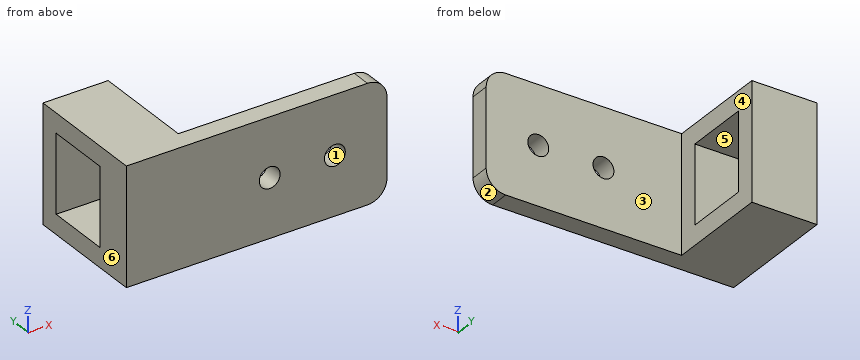
Autodesk Inventor part; units mm, degrees
ref_plane "YZ Plane" through (0, 0, 0) normal (1, 0, 0) x (0, 1, 0)
ref_plane "XZ Plane" through (0, 0, 0) normal (0, 1, 0) x (-1, 0, 0)
ref_plane "XY Plane" through (0, 0, 0) normal (0, 0, 1) x (1, 0, 0)
sketch "Sketch1" plane through (0, 0, 0) normal (1, 0, 0) x (0, 1, 0)
  line L0 (0, 0) -> (10, 0)
  line L1 (10, 0) -> (10, -12)
  line L2 (10, -12) -> (0, -12)
  line L3 (0, -12) -> (0, 0)
  line L4 (13, 3) -> (-6, 3)
  line L5 (-6, 3) -> (-6, -15)
  line L6 (-6, -15) -> (13, -15)
  line L7 (13, -15) -> (13, 3)
  dimension "d0" = 10
  dimension "d1" = 12
  dimension "d2" = 3
  dimension "d3" = 3
  dimension "d4" = 6
  dimension "d5" = 3
extrude "Extrusion1" add sketch "Sketch1" along normal blind 10
sketch "Sketch2" plane through (10, 0, 0) normal (1, 0, 0) x (0, 0, -1)
  line L0 (15, -6) -> (15, 13) construction
  line L1 (-3, -6) -> (15, -6) construction
  line L2 (-3, 13) -> (-3, -6) construction
  line L3 (15, -6) -> (15, 13)
  line L4 (-3, -6) -> (15, -6)
  line L5 (15, -6) -> (15, -3)
  line L6 (15, -3) -> (-3, -3)
  line L7 (-3, -3) -> (-3, -6)
  point P0 (0, 0)
  dimension "d8" = 3
extrude "Extrusion2" add sketch "Sketch2" along normal blind 30
sketch "Sketch3" plane through (10, -3, 3) normal (0, 1, 0) x (1, 0, 0)
  circle A0 centre (12, 9) radius 1.6
  circle A1 centre (22, 9) radius 1.6
  line L0 (0, 18) -> (30, 18)
  line L1 (0, 0) -> (30, 0)
  line L2 (30, 18) -> (30, 0)
  point P0 (-10, 3)
  dimension "d11" = 3.2
  dimension "d12" = 3.2
  dimension "d13" = 9
  dimension "d14" = 9
  dimension "d15" = 8
  dimension "d16" = 10
extrude "Extrusion3" cut sketch "Sketch3" against normal through all
fillet "Fillet1" radius 3 2 edges at (40, -4.5, 3) (40, -4.5, -15)
equation "\"d3\" = d2"
equation "\"d4\" = 2 * d2"
equation "\"d5\" = d2"
properties part number "Wheel Holder Rev 2"
Part model, mm, in its own coordinate system. Face numbers are marked on the shaded views. A direction names the side the tool comes from. Coordinates: 2 decimals unless noted, no trailing zeros. Loops run counter-clockwise (first coordinate to the right, second up) from the corner with the lowest first, then second, coordinate; pieces in that order, holes last. Notation, with made-up numbers: (84, 42) - (104, 42) arc R29 cw to (104, 70) - close; hole circle Ø8 at (82.25, 52.5). An arc over 180 degrees is marked (long way). Write each question's results on one line, items separated by ' | '. Start each with the question number.
Q1. Probe line 1 along X through (y, z) = (-5.3, -6); line 2 along Y through (x, z) = (9.5, -1); line 3 along Z through (x, y) = (32, -4.45). List the from-to ranges inside material, lowest first.
Q2. Which spindle directions (+Z, -Z, +X, -X, +Y, -Y) get a long thin tool onto all of the face, cutting with end or side? Do the marked faces 4, 5 and 6. Say none if no direction does.
Q3. Two-plate mould, pull along X, no slides. Class the marked faces 1, 2 and 3: +X half, -X half, draft (parallel to the pull), parting line (faces both ways), or undercut.
Q4. Drop flat-ended pins along their axis: pin 1 Ø8 at (y, z) = (4, 0) entering from +X; pin 2 Ø1.9 at (x, z) = (22, -6) entering from +Y; pin 3 Ø1 at (x, z) = (29, 0) entering from +Y. Give the stop position or say it passes through.
Q5. Slice it at B-B on y = 3.5. Give the cut face in (x, z).
Q6. Slice it at D-D on x = 32. Give the cut face in (y, z).
Q7. Slice it at C-C on y = -4. Give the cut face in (x, z), and give its area (3 significant figures).
Q8. Slice it at A-A on z = -6. Give the cut face in (x, y), and give its area (3 significant figures).
Answer:
1) line 1: x = 0 to 20.4, 23.6 to 30.4, 33.6 to 40 | line 2: y = -6 to 0, 10 to 13 | line 3: z = -15 to -7.6, -4.4 to 3
2) face 4: +Z, -Z, +X, +Y | face 5: +X, -X | face 6: +Z, -Z, -X, +Y, -Y
3) face 1: undercut | face 2: +X half | face 3: draft
4) pin 1: stops at x = 10 | pin 2: passes through | pin 3: stops at y = -3
5) outline: (0, -15) - (10, -15) - (10, -12) - (0, -12) - close; (0, 0) - (10, 0) - (10, 3) - (0, 3) - close
6) outline: (-6, -15) - (-3, -15) - (-3, -7.6) - (-6, -7.6) - close; (-6, -4.4) - (-3, -4.4) - (-3, 3) - (-6, 3) - close
7) outline: (0, -15) - (37, -15) arc R3 ccw to (40, -12) - (40, 0) arc R3 ccw to (37, 3) - (0, 3) - close; hole circle Ø3.2 at (22, -6); hole circle Ø3.2 at (32, -6) | area: 700 mm2
8) outline: (0, -6) - (20.4, -6) - (20.4, -3) - (10, -3) - (10, 0) - (0, 0) - close; (0, 10) - (10, 10) - (10, 13) - (0, 13) - close; (23.6, -6) - (30.4, -6) - (30.4, -3) - (23.6, -3) - close; (33.6, -6) - (40, -6) - (40, -3) - (33.6, -3) - close | area: 161 mm2
